Solid Edge part; units mm, degrees
sketch "Sketch1" plane through (0, 0, 8) normal (0, 0, 1) x (1, 0, 0)
  circle A0 centre (0, 0) radius 21
  circle A1 centre (0, 0) radius 12
  circle A2 centre (11.3137, 11.3137) radius 1.7
  circle A3 centre (-11.3137, 11.3137) radius 1.7
  circle A4 centre (-11.3137, -11.3137) radius 1.7
  circle A5 centre (11.3137, -11.3137) radius 1.7
extrude "ExtrudedProtrusion_1" add sketch "Sketch1" along normal blind 4
sketch "Sketch2" plane through (0, 0, 8) normal (0, 0, 1) x (1, 0, 0)
  line L0 (12, -12) -> (88, -12)
  line L1 (88, -12) -> (88, 12)
  line L2 (88, 12) -> (12, 12)
  line L3 (12, 12) -> (12, -12)
extrude "ExtrudedProtrusion_2" add sketch "Sketch2" along normal blind 4
sketch "Sketch3" plane through (0, 0, 8) normal (0, 0, 1) x (1, 0, 0)
  line L0 (72, -49) -> (128, -49)
  line L1 (128, -49) -> (128, 24)
  line L2 (128, 24) -> (72, 24)
  line L3 (72, 24) -> (72, -49)
  circle A0 centre (77, -43) radius 1.7
  circle A1 centre (123, -43) radius 1.7
  circle A2 centre (77, 18) radius 1.7
  circle A3 centre (123, 18) radius 1.7
extrude "ExtrudedProtrusion_3" add sketch "Sketch3" along normal blind 4
Check sheet for the modelled part. Datum: model origin and axes. Units: mm. A direction names the side the tool comes from. Round coordinates to 2 decimals unless told otherwise and drop trailing zeros. Order: outer loops, then holes, each group sorted by start corner. A loop starts at its lowest first (then second) coordinate and runs counter-clockwise, first axis right, second up. Notation, with made-up numbers: M 87,-27.75 L 119,-27.75 A27 cw 119,-9.75 Z; hole C 65.5,31.5 d2. An arc over 180 degrees is marked long. One line per item, written item: value. Start each with the question number.
1. Gauge pin test, flat ends, axial feed: P1, Ø1.2, axis at y = -27, z = 11, coming from the -X side; P2, Ø2, axis at x = 34, z = 9.5, coming from the -Y side; P3, Ø1, axis at x = 12.5, z = 9, coming from the +Y side. Record the tip position at first contact, or that the pin passes through.
2. Release check for a two-part mould opening along X. For faces 1 (the flat face through (100, 24, 10)), 2 (the flat face through (128, -13, 10)), 3 (the cylindrical face through (9.71, 11.88, 9.97)) record: released by +X, released by -X, zero draft, split by the parting line, or undercut.
3. Section check B-B on x = 0. Enter the section's corners in (y, z), and give its area (3 significant figures).
4. Scan lines: line 1 along Y through (x, z) = (123, 10.7); line 2 along Y through (x, z) = (0, 9.9); line 3 along Y through (x, z) = (76.5, 10.25). Record each from-to range of solid material in increasing order.
5. Section check A-A on y = 0. Enter the section's corners in (x, z), and give its area (3 significant figures).
6. Section check C-C on x = 77. Enter the section's corners in (y, z), and give its area (3 significant figures).
7. Section check D-D on z = 9.65. Give the number of separate pieces and of enclosed holes in the cut face, and give its area (3 significant figures).
8. Access from +Z, -Z, +X, -X, +Y, -Y to the whole of each face (thin tool, end or side, straight path). Record for faces 4 (the cylindrical face through (75.3, 17.93, 9.97)), 5 (the flat face through (72, 18, 10)), 6 (the flat face through (72, -30, 10)).
Results found:
1. P1: x = 72
1. P2: y = -12
1. P3: y = 17.23
2. face 1: zero draft
2. face 2: released by +X
2. face 3: undercut
3. outline: M -21,8 L -12,8 L -12,12 L -21,12 Z; M 12,8 L 21,8 L 21,12 L 12,12 Z
3. area: 72.0 mm^2
4. line 1: -49 to -44.7, -41.3 to 16.3, 19.7 to 24
4. line 2: -21 to -12, 12 to 21
4. line 3: -49 to -44.62, -41.38 to 16.38, 19.62 to 24
5. outline: M -21,8 L -12,8 L -12,12 L -21,12 Z; M 12,8 L 128,8 L 128,12 L 12,12 Z
5. area: 500 mm^2
6. outline: M -49,8 L -44.7,8 L -44.7,12 L -49,12 Z; M -41.3,8 L 16.3,8 L 16.3,12 L -41.3,12 Z; M 19.7,8 L 24,8 L 24,12 L 19.7,12 Z
6. area: 265 mm^2
7. separate pieces: 1
7. enclosed holes: 9
7. area: 6,200 mm^2
8. face 4: +Z, -Z
8. face 5: +Z, -Z, +Y
8. face 6: +Z, -Z, -Y
